Work out the finished part from the listing and answer in its coordinate system (mm). A direction names the side the tool comes from. Give positions to 0.01 mm unless a question says otherwise; leave off trailing zeros. Loops run counter-clockwise (first coordinate to the right, second up) from the corner with the lowest first, then second, coordinate; pieces in that order, holes last. Notation, with made-up numbers: (-0.5, 60) - (34.5, 60) arc R21 cw to (34.5, 79) - close; hole circle Ø10 at (47.25, 9.5). An arc over 180 degrees is marked (long way). Use one line per item in the form item = value. Start each with the question number.
Autodesk Inventor part; units mm, degrees
ref_plane "YZ Plane" through (0, 0, 0) normal (1, 0, 0) x (0, 1, 0)
ref_plane "XZ Plane" through (0, 0, 0) normal (0, 1, 0) x (-1, 0, 0)
ref_plane "XY Plane" through (0, 0, 0) normal (0, 0, 1) x (1, 0, 0)
sketch "スケッチ1" plane through (0, 0, 0) normal (0, 0, 1) x (1, 0, 0)
  circle A0 centre (0, 0) radius 6
  circle A1 centre (0, 0) radius 3
  circle A2 centre (0, 0) radius 6.8
  circle A3 centre (0, 0) radius 5.5
  circle A4 centre (0, 0) radius 3.5
  dimension "d0" = 12
  dimension "d1" = 6
  dimension "d4" = 0.8
  dimension "d6" = 0.5
  dimension "d7" = 0.5
extrude "押し出し1" add sketch "スケッチ1" along normal blind 0.8 contours A2
extrude "押し出し2" add sketch "スケッチ1" along normal blind 4 contours A0 | A4
extrude "押し出し3" add sketch "スケッチ1" along normal blind 3.5 contours A3
extrude "押し出し5" cut sketch "スケッチ1" along normal blind 0.5 contours A3
properties part number "ベアリングフランジ6-12"
1) Determine the mould class of faces 1 (the flat face through (4, 0, 3.5)), 2 (the flat face through (4, -5, 0.8)), 3 (the cylindrical face through (-6, 0, 2)) for opening direction X: released by +X, released by -X, zero draft, split by the parting line, or undercut.
2) A cutting plane is placed at A-A (x = 0). Give the vertices of the cut face in (y, z), plus the area to 3 significant figures.
3) A flat-ended cylindrical pin translates along its axis: pin 1 Ø2 at (x, z) = (-4.5, 3.5) entering from -Y. Find the tip coordinate at first contact, or state that the pin passes through.
4) Find the intervals of material crossed by probe 1 along Y at (x, z) = (0, 0.1); probe 2 along Y at (x, z) = (0, 3.65); probe 3 along Y at (x, z) = (0, 1.3), in increasing order.
5) A cutting plane is placed at B-B (y = -2.75). Give the vertices of the cut face in (x, z).
6) A cutting plane is placed at C-C (z = 2.9). Give the vertices of the cut face in (x, y).
7) A cutting plane is placed at D-D (y = 5). Give the vertices of the cut face in (x, z).
8) A tool of negligible diameter and unlimited length cuts with its end or side. For faces 4 (the cylindrical face through (3.233, 1.341, 3.746)), 5 (the flat face through (3, 1, 0)), 6 (the cylindrical face through (-1.19, 5.37, 0.25)), from which of +Z, -Z, +X, -X, +Y, -Y can it reach the whole face along a straight path? Write none if from no direction.
Answer sheet:
q1.face_1 = undercut
q1.face_2 = zero draft
q1.face_3 = split by the parting line
q2.outline = (-6.8, 0) - (-5.5, 0) - (-5.5, 0.5) - (-3.5, 0.5) - (-3.5, 0) - (-3, 0) - (-3, 4) - (-3.5, 4) - (-3.5, 3.5) - (-5.5, 3.5) - (-5.5, 4) - (-6, 4) - (-6, 0.8) - (-6.8, 0.8) - close; (3, 0) - (3.5, 0) - (3.5, 0.5) - (5.5, 0.5) - (5.5, 0) - (6.8, 0) - (6.8, 0.8) - (6, 0.8) - (6, 4) - (5.5, 4) - (5.5, 3.5) - (3.5, 3.5) - (3.5, 4) - (3, 4) - close
q2.area = 21.3 mm²
q3.pin_1 = -4.87
q4.probe_1 = -6.8 to -5.5, -3.5 to -3, 3 to 3.5, 5.5 to 6.8
q4.probe_2 = -6 to -5.5, -3.5 to -3, 3 to 3.5, 5.5 to 6
q4.probe_3 = -6 to -3, 3 to 6
q5.outline = (-6.22, 0) - (-4.76, 0) - (-4.76, 0.5) - (-2.17, 0.5) - (-2.17, 0) - (-1.2, 0) - (-1.2, 4) - (-2.17, 4) - (-2.17, 3.5) - (-4.76, 3.5) - (-4.76, 4) - (-5.33, 4) - (-5.33, 0.8) - (-6.22, 0.8) - close; (1.2, 0) - (2.17, 0) - (2.17, 0.5) - (4.76, 0.5) - (4.76, 0) - (6.22, 0) - (6.22, 0.8) - (5.33, 0.8) - (5.33, 4) - (4.76, 4) - (4.76, 3.5) - (2.17, 3.5) - (2.17, 4) - (1.2, 4) - close
q6.outline = circle Ø12 at (0, 0); hole circle Ø6 at (0, 0)
q7.outline = (-4.61, 0) - (-2.29, 0) - (-2.29, 0.5) - (2.29, 0.5) - (2.29, 0) - (4.61, 0) - (4.61, 0.8) - (3.32, 0.8) - (3.32, 4) - (2.29, 4) - (2.29, 3.5) - (-2.29, 3.5) - (-2.29, 4) - (-3.32, 4) - (-3.32, 0.8) - (-4.61, 0.8) - close
q8.face_4 = +Z
q8.face_5 = -Z, +X, -X, +Y, -Y
q8.face_6 = -Z
